```python
from build123d import *

# Parameters (mm, degrees)
BOSS_EXTRUDE1_DEPTH     = 38.1
SKETCH3_R               = 2.286
CUT_EXTRUDE2_DEPTH      = 6.08
SKETCH4_W               = 10.922
SKETCH4_H               = 7.62
CUT_EXTRUDE3_DEPTH      = 6.08
CUT_EXTRUDE3_DEPTH_BACK = 6.08
SKETCH7_R               = 2.286
CUT_EXTRUDE4_DEPTH      = 31.48


with BuildPart() as part:
    # Sketch1 → Boss-Extrude1 (new body)
    with BuildSketch(Plane.XY):
        with BuildLine():
            Line((0, 0), (0, 5.08))
            Line((0, 5.08), (17.78, 5.08))
            ThreePointArc((17.78, 5.08), (26.452102448, 8.672102448), (22.86, 0))
            Line((22.86, 0), (0, 0))
        make_face()
    extrude(amount=BOSS_EXTRUDE1_DEPTH)

    # Sketch3 → Cut-Extrude2 (cut, through all)
    with BuildSketch(Plane(origin=(0, 5.08, 0), x_dir=(1, 0, 0), z_dir=(0, 1, 0))):
        with Locations((6.477, -10.414)):
            Circle(SKETCH3_R)
        with Locations((6.477, -27.686)):
            Circle(SKETCH3_R)
    extrude(amount=-CUT_EXTRUDE2_DEPTH, mode=Mode.SUBTRACT)

    # Sketch4 → Cut-Extrude3 (cut, two sides)
    with BuildSketch(Plane(origin=(0, 5.08, 0), x_dir=(1, 0, 0), z_dir=(0, 1, 0))) as cut_extrude3_sk:
        with Locations((22.479, -3.81)):
            Rectangle(SKETCH4_W, SKETCH4_H)
        with Locations((22.479, -34.29)):
            Rectangle(SKETCH4_W, SKETCH4_H)
        with Locations((22.479, -19.05)):
            Rectangle(SKETCH4_W, SKETCH4_H)
    extrude(amount=CUT_EXTRUDE3_DEPTH, mode=Mode.SUBTRACT)
    extrude(cut_extrude3_sk.sketch, amount=-CUT_EXTRUDE3_DEPTH_BACK, mode=Mode.SUBTRACT)

    # Sketch7 → Cut-Extrude4 (cut, through all)
    with BuildSketch(Plane.XY.offset(30.48)):
        with Locations((22.86, 5.08)):
            Circle(SKETCH7_R)
    extrude(amount=-CUT_EXTRUDE4_DEPTH, mode=Mode.SUBTRACT)


solid = part.part
```
CAD build for the part. Positions are in the model's coordinates, mm. A direction names the side the tool comes from. Coordinates: 2 decimals unless noted, no trailing zeros. Write each loop counter-clockwise with the first axis right and the second up, starting at its lowest first coordinate (ties: lowest second). Pieces come first, ordered by that corner, then holes.
(1) Cut at D-D, the plane y = 1.25. List the corners of the cut face in (x, z).
(2) Drill centre lines: probe 1 along Z at (x, y) = (17.5, 5); probe 2 along Y at (x, z) = (22.86, 9.75); probe 3 along Y at (x, z) = (11.75, 8). Where is each one in solid material? Low to high.
(3) Cut at A-A, the plane z = 11.5. List the corners of the cut face in (x, y).
(4) Cut at B-B, the plane x = 19. List the corners of the cut face in (y, z), and give its area (3 significant figures).
(5) Flat gauge pins, fed straight in: pin 1 (3 mm diameter, centred on x = 24, y = 4.5, fed in from +Z); pin 2 (2.5 mm diameter, centred on y = 1.5, z = 35.5, fed in from +X); pin 3 (5 mm diameter, centred on x = 23.5, y = 5, fed in from -Z). Where does each tip first touch, or does it go through?
(6) Cut at C-C, the plane y = 8.5. List the corners of the cut face in (x, z).
(7) 3-axis set-ups, long thin cutter, end or side, ignore diameter. For faces 1 (the face through (21, 3, 30.48)), 2 (the face through (26.33, 8.79, 26.62)), 3 (the face through (9, 5.08, 19)), 4 (the face through (17.018, 3, 19)), 5 (the face through (17.018, 3, 4)): which of +Z, -Z, +X, -X, +Y, -Y reach the whole face in a straight line?
(8) Two-plate mould, pull along Y, no slides. Class faces 6 (the face through (20.576, 5.181, 26.723)), 7 (the face through (21, 3, 22.86)), 8 (the face through (26.33, 8.79, 11.38)): +Y half, -Y half, draft (parallel to the pull), parting line (faces both ways), or undercut.
Geometry says:
1. outline: (0, 0) - (17.02, 0) - (17.02, 7.62) - (26.2, 7.62) - (26.2, 15.24) - (17.02, 15.24) - (17.02, 22.86) - (26.2, 22.86) - (26.2, 30.48) - (17.02, 30.48) - (17.02, 38.1) - (0, 38.1) - close; hole circle Ø4.57 at (6.48, 10.41); hole circle Ø4.57 at (6.48, 27.69)
2. probe 1: z = 7.62 to 15.24, 22.86 to 30.48
2. probe 2: y = 0 to 2.79, 7.37 to 10.16
2. probe 3: y = 0 to 5.08
3. outline: (0, 0) - (4.47, 0) - (4.47, 5.08) - (0, 5.08) - close; (8.49, 0) - (22.86, 0) arc R5.08 ccw (long way) to (17.78, 5.08) - (8.49, 5.08) - close; hole circle Ø4.57 at (22.86, 5.08)
4. outline: (0, 7.62) - (8.38, 7.62) - (8.38, 15.24) - (0, 15.24) - close; (0, 22.86) - (8.38, 22.86) - (8.38, 30.48) - (0, 30.48) - close
4. area: 128 mm2
5. pin 1: stops at z = 30.48
5. pin 2: stops at x = 17.02
5. pin 3: stops at z = 7.62
6. outline: (19.1, 7.62) - (26.62, 7.62) - (26.62, 15.24) - (19.1, 15.24) - close; (19.1, 22.86) - (26.62, 22.86) - (26.62, 30.48) - (19.1, 30.48) - close
7. face 1: +Z, +X, +Y, -Y
7. face 2: +Z, -Z
7. face 3: +Z, -Z, -X, +Y
7. face 4: +X, +Y, -Y
7. face 5: -Z, +X, +Y, -Y
8. face 6: undercut
8. face 7: draft
8. face 8: parting line
